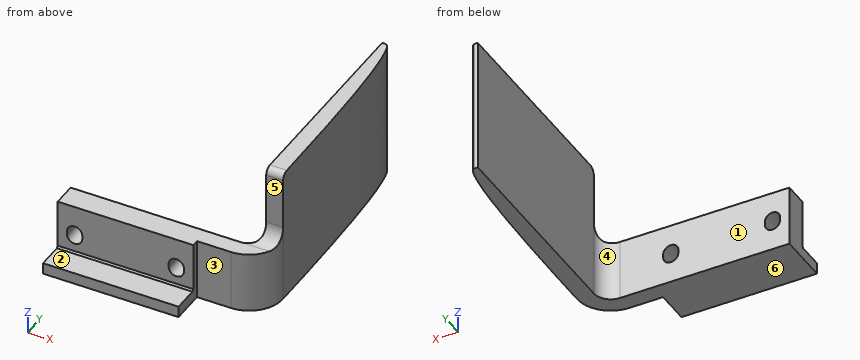
Autodesk Inventor part; units mm, degrees
ref_plane "YZ Plane" through (0, 0, 0) normal (1, 0, 0) x (0, 1, 0)
ref_plane "XZ Plane" through (0, 0, 0) normal (0, 1, 0) x (-1, 0, 0)
ref_plane "XY Plane" through (0, 0, 0) normal (0, 0, 1) x (1, 0, 0)
sketch "スケッチ1" plane through (0, 0, 0) normal (0, 0, 1) x (1, 0, 0)
  line L0 (0, 0) -> (0, 5)
  line L1 (0, 5) -> (50, 5)
  line L2 (55, 10) -> (55, 73)
  line L3 (55, 73) -> (60, 73)
  line L4 (60, 73) -> (60, 10)
  line L5 (50, 0) -> (0, 0)
  arc A0 (50, 0) -> (60, 10) centre (50, 10) ccw
  line L6 (0, 0) -> (50, 0)
  line L7 (40, 0) -> (40, -2)
  line L8 (40, -2) -> (0, -2)
  line L9 (0, -2) -> (0, 0)
  arc A1 (50, 5) -> (55, 10) centre (50, 10) ccw
  point P0 (60, 0)
  point P1 (55, 5)
  point P2 (40, 0)
  dimension "d0" = 55
  dimension "d1" = 73
  dimension "d2" = 5
  dimension "d3" = 5
  dimension "d5" = 10
  dimension "d34" = 2
  dimension "d35" = 40
  dimension "d58" = 5
extrude "押し出し1" add sketch "スケッチ1" along normal mid plane 18
sketch "スケッチ2" plane through (0, 5, 9) normal (0, 1, 0) x (1, 0, 0)
  line L0 (50, 0) -> (0, 0)
  line L1 (0, 18) -> (0, 0)
  point P0 (5, 9)
  point P1 (35, 9)
  dimension "d8" = 30
  dimension "d59" = 9
  dimension "d60" = 5
hole "穴1" at (5, 5, 0) at (35, 5, 0) direction (0, -1, 0) diameter 4.5 end through all
sketch "スケッチ3" plane through (0, 0, 9) normal (0, 0, 1) x (1, 0, 0)
  line L0 (60, 10) -> (60, 73)
  line L1 (60, 73) -> (55, 73)
  line L2 (55, 73) -> (55, 10)
  line L3 (50, 5) -> (0, 5)
  line L4 (0, 5) -> (0, -2)
  arc A0 (50, 0) -> (60, 10) centre (50, 10) ccw
  line L5 (0, -2) -> (40, -2)
  line L6 (40, -2) -> (40, 0)
  line L7 (40, 0) -> (50, 0)
  line L8 (60, 10) -> (55, 10)
  line L9 (55, 73) -> (55, 10)
  arc A1 (50, 5) -> (55, 10) centre (50, 10) ccw
  point P0 (55, 6)
  point P1 (55, 10)
extrude "押し出し2" add sketch "スケッチ3" along normal blind 22 contours L8 L2 L1 L0
sketch "スケッチ4" plane through (0, -2, 9) normal (0, -1, 0) x (1, 0, 0)
  line L0 (0, -18) -> (40, -18)
  line L1 (40, -18) -> (40, -14.653)
  line L2 (40, -14.653) -> (0, -14.653)
  line L3 (0, -14.653) -> (0, -18)
  point P0 (0, -9)
  dimension "d20" = 40
  dimension "d21" = 3.347
extrude "押し出し3" add sketch "スケッチ4" along normal blind 8
chamfer "面取り1" distance 0.5 angle 45 1 edges at (20, -2, -5.653)
sketch "スケッチ6" plane through (0, 5, -9) normal (0, 1, 0) x (1, 0, 0)
  circle A0 centre (5, -9) radius 2.25
  circle A1 centre (35, -9) radius 2.25
  line L0 (5, -9.5) -> (5, -8.5) construction
  line L1 (7.25, -9.5) -> (7.25, -8.5)
  line L2 (2.75, -8.5) -> (2.75, -9.5)
  arc A2 (2.75, -9.5) -> (7.25, -9.5) centre (5, -9.5) ccw
  arc A3 (7.25, -8.5) -> (2.75, -8.5) centre (5, -8.5) ccw
  line L3 (35, -9.5) -> (35, -8.5) construction
  line L4 (32.75, -9.5) -> (32.75, -8.5)
  line L5 (37.25, -8.5) -> (37.25, -9.5)
  arc A4 (32.75, -9.5) -> (37.25, -9.5) centre (35, -9.5) ccw
  arc A5 (37.25, -8.5) -> (32.75, -8.5) centre (35, -8.5) ccw
  point P0 (0, -9)
  dimension "d37" = 1
  dimension "d38" = 1
extrude "押し出し5" cut sketch "スケッチ6" against normal blind 18
sketch "スケッチ5" plane through (0, 0, 31) normal (0, 0, 1) x (1, 0, 0)
  line L0 (55, 73) -> (60, 73)
  line L1 (60, 73) -> (60, 10)
  line L2 (55, 73) -> (55, 10)
  line L3 (60, 10) -> (60, 73) construction
  line L4 (60, 73) -> (56, 73) construction
  spline S0 degree 2 poles (60, 10) (60, 73) (56, 73) knots 1 1 1 2 2 2
  line L5 (60, 73) -> (55, 73)
  point P0 (0, 0)
  point P1 (55, 13)
  point P2 (55, 8)
  dimension "d30" = 1
extrude "押し出し4" cut sketch "スケッチ5" against normal through all
fillet "フィレット10" radius 2 1 edges at (57.5, 10, 31)
fillet "フィレット11" radius 5 1 edges at (57.5, 10, 9)
properties part number "base49"
Design review of the part built by this model. Coordinates are the model's own, in mm. Face numbers are marked on the shaded views. A direction names the side the tool comes from. Coordinates: 2 decimals unless noted, no trailing zeros. Write each loop counter-clockwise with the first axis right and the second up, starting at its lowest first coordinate (ties: lowest second). Pieces come first, ordered by that corner, then holes. Notation, with made-up numbers: M 33.25,-33 L 63.25,-33 A20 cw 63.25,-14 Z; hole C -35.75,36 d7. An arc over 180 degrees is marked long. Answer as a JSON object with one key per item and string values.
Item 1: Add section A-A, the plane x = 5. Give the boundary of the cut face in (y, z).
Outcome:
{"outline": "M -10,-9 L 5,-9 L 5,-2.75 L -2,-2.75 L -2,-5.15 L -2.5,-5.65 L -10,-5.65 Z; M -2,2.75 L 5,2.75 L 5,9 L -2,9 Z"}
Item 2: Wall thickness on probe 1 along Z at (x, y) = (39, -3); probe 2 along Y at (x, z) = (25, 6); probe 3 along Y at (x, z) = (48, -1.5): over which ranges is each line inside the solid? List them lowest first.
Outcome:
{"probe 1": "-9 to -5.65", "probe 2": "-2 to 5", "probe 3": "0 to 5"}
Item 3: Draft analysis for pull direction Y (two halves, no side actions). For the marked faces 4, 5 and 6, state which applies: pulls with the +Y half, pulls with the -Y half, needs draft (parallel to the pull), parting line crosses it, or undercut.
Outcome:
{"face 4": "pulls with the +Y half", "face 5": "pulls with the -Y half", "face 6": "needs draft"}
Item 4: Machinability: for the marked faces 1, 2 and 3, which of the approach directions +Z, -Z, +X, -X, +Y, -Y give a long, thin tool a straight path to every point of the face, cutting with its end or side? Answer none if there is none.
Outcome:
{"face 1": "+Z, -Z, -X, +Y", "face 2": "+Z, +X, -X, -Y", "face 3": "+Z, -Z, +X, -Y"}
Item 5: Insertion check: pin 1 Ø4 at (y, z) = (24, 10.5) entering from -X; pin 2 Ø8 at (x, y) = (24.5, -5.5) entering from +Z; pin 3 Ø3 at (x, z) = (9.5, -5) entering from +Y. Each pin has a flat end and moves straight along its axis. Give the tip position at first contact, or say it passes through.
Outcome:
{"pin 1": "x = 55", "pin 2": "z = 9", "pin 3": "y = 5"}
